Check sheet for the modelled part. Datum: model origin and axes. Units: mm. Face numbers are marked on the shaded views. A direction names the side the tool comes from. Coordinates: 2 decimals unless noted, no trailing zeros. Loops run counter-clockwise (first coordinate to the right, second up) from the corner with the lowest first, then second, coordinate; pieces in that order, holes last.
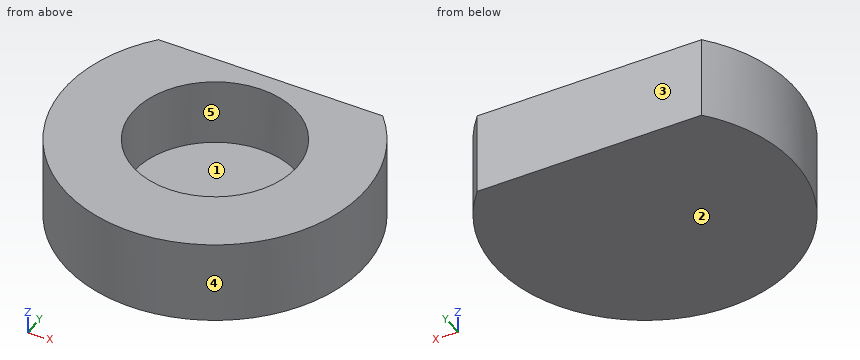
```python
from build123d import *

# Parameters (mm, degrees)
BOX002_W               = 10
BOX002_H               = 35
BOX002_DEPTH           = 15
CYLINDER015_R          = 9.8
CYLINDER015_DEPTH      = 110
CYLINDER014_R          = 18
CYLINDER014_DEPTH      = 10
CUT003_PLACEMENT_ANGLE = 90


with BuildPart() as cube002:
    # Box002 → Box002 (new body)
    with BuildSketch(Plane(origin=(-22, -18.5, -3), x_dir=(1, 0, 0), z_dir=(0, 0, 1))):
        with Locations((5, 17.5)):
            Rectangle(BOX002_W, BOX002_H)
    extrude(amount=BOX002_DEPTH)


with BuildPart() as main_axis002:
    # Cylinder015 → Cylinder015 (new body)
    with BuildSketch(Plane.XY):
        Circle(CYLINDER015_R)
    extrude(amount=CYLINDER015_DEPTH)


with BuildPart() as main_axis_holder:
    # Cylinder014 → Cylinder014 (new body)
    with BuildSketch(Plane.XY.offset(-2)):
        Circle(CYLINDER014_R)
    extrude(amount=CYLINDER014_DEPTH)

    # Cut002: cut main_axis002
    add(main_axis002.part, mode=Mode.SUBTRACT)

    # Cut003: cut Cube002
    add(cube002.part, mode=Mode.SUBTRACT)


with BuildPart() as main_axis_holder_1:
    # Cut003 placement: moved
    add(main_axis_holder.part.rotate(Axis((0, 0, 0), (0, 0, -1)), CUT003_PLACEMENT_ANGLE))


solid = main_axis_holder_1.part
```
1) Mould release check, pull along X, two halves, no side actions. Record for the marked faces 3, 4 and 5: +X half, -X half, draft (parallel to the pull), parting line (faces both ways), or undercut.
Answer sheet:
face 3: draft
face 4: parting line
face 5: undercut
2) Section check A-A on x = 0. Enter the section's corners in (y, z).
Answer sheet:
outline: (-18, -2) - (12, -2) - (12, 8) - (9.8, 8) - (9.8, 0) - (-9.8, 0) - (-9.8, 8) - (-18, 8) - close
3) Section check D-D on x = 15.5. Enter the section's corners in (y, z), plus the area to 3 significant figures.
Answer sheet:
outline: (-9.15, -2) - (9.15, -2) - (9.15, 8) - (-9.15, 8) - close
area: 183 mm2
4) Set-up check for the marked faces 1 and 2: record each of +Z, -Z, +X, -X, +Y, -Y from which the full face is reachable in a straight line by a thin tool's end or side.
Answer sheet:
face 1: +Z
face 2: -Z, +X, -X, +Y, -Y
5) Depth check by flat-ended pin: pin 1 (1.5 mm diameter, centred on y = 6, z = 3, fed in from -X); pin 2 (1.5 mm diameter, centred on x = 1, y = 0.5, fed in from +Z); pin 3 (6 mm diameter, centred on x = 11, z = 2, fed in from -Y). Enter the tip coordinate at first touch or a pass-through.
Answer sheet:
pin 1: stops at x = -17.22
pin 2: stops at z = 0
pin 3: stops at y = -16.12
6) Section check C-C on z = 5.5. Enter the section's corners in (x, y), plus the area to 3 significant figures.
Answer sheet:
outline: (-13.42, 12) arc R18 ccw (long way) to (13.42, 12) - close; hole circle Ø19.6 at (0, 0)
area: 605 mm2
7) Section check B-B on y = -6.5. Enter the section's corners in (x, z), plus the area to 3 significant figures.
Answer sheet:
outline: (-16.79, -2) - (16.79, -2) - (16.79, 8) - (7.33, 8) - (7.33, 0) - (-7.33, 0) - (-7.33, 8) - (-16.79, 8) - close
area: 218 mm2
8) Scan lines: line 1 (X direction, y = 0, z = 3.5); line 2 (Z direction, x = 5.5, y = -4); line 3 (X direction, y = -3, z = 6.75). Record each from-to range of solid material in increasing order.
Answer sheet:
line 1: x = -18 to -9.8, 9.8 to 18
line 2: z = -2 to 0
line 3: x = -17.75 to -9.33, 9.33 to 17.75
